The model under review builds one solid part; all positions refer to its coordinate system, in mm. A direction names the side the tool comes from. Give positions to 0.01 mm unless a question says otherwise; leave off trailing zeros. Loops run counter-clockwise (first coordinate to the right, second up) from the corner with the lowest first, then second, coordinate; pieces in that order, holes last. Notation, with made-up numbers: (81.5, 84) - (130.5, 84) arc R30 ccw to (130.5, 115) - close; hole circle Ø5 at (-35.75, 10). An arc over 180 degrees is marked (long way). Answer as a JSON object with one key per item and string values.
from build123d import *

# Parameters (mm, degrees)
F0_W     = 18
F0_H     = 18
F1_DEPTH = 10
F2_W     = 15.5
F2_H     = 7.1
F3_DEPTH = 16
F4_R     = 5.08
F5_R     = 5.08
F6_R     = 1.27


with BuildPart() as f1:
    # F0 (on Top) → F1 (new body)
    with BuildSketch(Plane.XY):
        Rectangle(F0_W, F0_H)
    extrude(amount=F1_DEPTH)

    # F2 (on face) → F3 (cut)
    with BuildSketch(Plane.XZ.offset(9)):
        with Locations((1.25, 4.95)):
            Rectangle(F2_W, F2_H)
    extrude(amount=-F3_DEPTH, mode=Mode.SUBTRACT)

    # F4
    f4_edges = [f1.edges().sort_by_distance(p)[0] for p in [
        (-9, 9, 5),
    ]]
    fillet(f4_edges, radius=F4_R)

    # F5
    f5_edges = [f1.edges().sort_by_distance(p)[0] for p in [
        (-6.5, 7, 4.95),
    ]]
    fillet(f5_edges, radius=F5_R)

    # F6
    f6_edges = [f1.edges().sort_by_distance(p)[0] for p in [
        (-9, -9, 5),
        (9, 9, 5),
        (9, -9, 0.7),
        (9, -9, 9.25),
    ]]
    fillet(f6_edges, radius=F6_R)


solid = f1.part
Q1. Consider section A-A, the plane z = 3.75. State the section outline as (x, y) points, plus the area to 3 significant figures.
Results:
{"outline": "(-9, -7.73) arc R1.27 ccw to (-7.73, -9) - (-6.5, -9) - (-6.5, 1.92) arc R5.08 cw to (-1.42, 7) - (9, 7) - (9, 7.73) arc R1.27 ccw to (7.73, 9) - (-3.92, 9) arc R5.08 ccw to (-9, 3.92) - close", "area": "75.3 mm^2"}
Q2. To check wall thickness, follow probe 1 along Z at (x, y) = (-1.25, 4); probe 2 along Y at (x, z) = (1, 4.5); probe 3 along X at (y, z) = (1.5, 6). State the ranges of each line that lie inside material, in increasing order. Write a range as [from, to].
Results:
{"probe 1": "z = [0, 1.4], [8.5, 10]", "probe 2": "y = [7, 9]", "probe 3": "x = [-9, -6.5]"}
Q3. Clearance check with flat-ended pins moving along their axes: pin 1 Ø4 at (x, z) = (2, 2) entering from -Y; pin 2 Ø1.5 at (y, z) = (-3, 2.5) entering from +X. State where each tip first meets the part, or that it passes through.
Results:
{"pin 1": "stops at y = -9", "pin 2": "stops at x = -6.5"}
Q4. Consider section C-C, the plane x = 0.25. State the section outline as (y, z) points, plus the area to 3 significant figures.
Results:
{"outline": "(-9, 0) - (9, 0) - (9, 10) - (-9, 10) - (-9, 8.5) - (7, 8.5) - (7, 1.4) - (-9, 1.4) - close", "area": "66.4 mm^2"}
Q5. Consider section B-B, the plane y = -6.5. State the section outline as (x, z) points.
Results:
{"outline": "(-9, 0) - (9, 0) - (9, 1.4) - (-6.5, 1.4) - (-6.5, 8.5) - (9, 8.5) - (9, 10) - (-9, 10) - close"}
Q6. The part is to be moulded in two halves that separate along Z. For faces 1 (the face through (4, 7, 5)), 2 (the face through (-9, -2, 5)), 3 (the face through (0, 0, 0)), say which applies: +Z half, -Z half, draft (parallel to the pull), parting line (faces both ways), or undercut.
Results:
{"face 1": "undercut", "face 2": "draft", "face 3": "-Z half"}
Q7. For faces 4 (the face through (8.618, -8.638, 0.71)), 5 (the face through (1, -1, 1.4)), list the 3-axis set-ups (+Z, -Z, +X, -X, +Y, -Y) from which the entire face can be reached by the end or side of a thin tool; tool diameter is ignored.
Results:
{"face 4": "+Z, -Z, +X, -Y", "face 5": "+X, -Y"}
